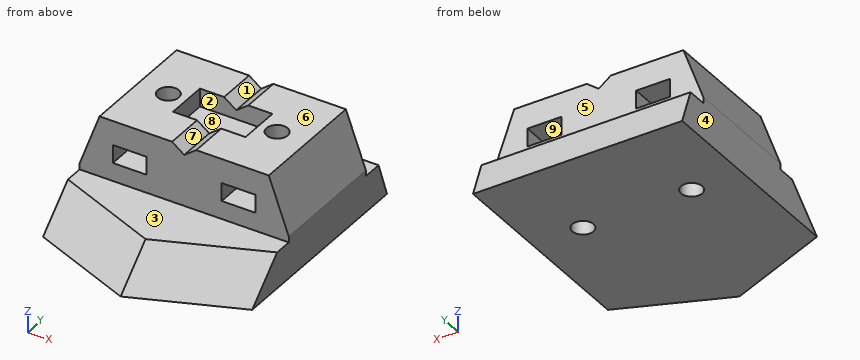
```python
from build123d import *

# Parameters (mm, degrees)
ESBO_O1_W                = 34.6
ESBO_O1_H                = 26
RESSALTO_EXTRUS_O1_DEPTH = 7
ESBO_O10_W               = 34.6
ESBO_O10_H               = 2.5
RESSALTO_EXTRUS_O4_DEPTH = 7
CHANFRO1_SIZE            = 7
CHANFRO2_SIZE2           = 7
CHANFRO2_SIZE            = 2.54779164
ESBO_O11_W               = 5.6
ESBO_O11_H               = 3
RESSALTO_EXTRUS_O5_DEPTH = 10
ESBO_O12_R               = 1.75
CORTE_EXTRUS_O1_DEPTH    = 20
ESBO_O13_W               = 34.6
ESBO_O13_H               = 5.5
ESBO_O13_H_2             = 18.393079324
CORTE_EXTRUS_O2_DEPTH    = 1
ESBO_O14_W               = 12
ESBO_O14_H               = 7
CORTE_EXTRUS_O3_DEPTH    = 3


with BuildPart() as part:
    # Esboço1 → Ressalto-extrusão1 (new body)
    with BuildSketch(Plane.XY):
        Rectangle(ESBO_O1_W, ESBO_O1_H)
    extrude(amount=RESSALTO_EXTRUS_O1_DEPTH)

    # Esboço10 → Ressalto-extrusão4 (add)
    with BuildSketch(Plane(origin=(0, 0, 0), x_dir=(-1, 0, 0), z_dir=(0, 0, -1))):
        Polygon((-17.3, -19.5), (0, -26.5), (17.3, -19.5), (17.3, -13), (-17.3, -13), align=None)
        with Locations((0, 14.25)):
            Rectangle(ESBO_O10_W, ESBO_O10_H)
    extrude(amount=-RESSALTO_EXTRUS_O4_DEPTH)

    # Chanfro1
    chanfro1_edges = [part.edges().sort_by_distance(p)[0] for p in [
        (8.65, -23, 7),
        (-8.65, -23, 7),
    ]]
    chamfer(chanfro1_edges, length=CHANFRO1_SIZE - 0.0001)  # a hair under: the kernel refuses the full size

    # Chanfro2
    chanfro2_edges = [part.edges().sort_by_distance(p)[0] for p in [
        (0, 15.5, 7),
    ]]
    chanfro2_side = [part.faces().sort_by_distance(p)[0] for p in [
        (0, 15.449044167, 7),
    ]]
    chamfer(chanfro2_edges, length=CHANFRO2_SIZE - 0.0001, length2=CHANFRO2_SIZE2 - 0.0001, reference=chanfro2_side[0])  # a hair under: the kernel refuses the full size

    # Esboço11 → Ressalto-extrusão5 (add, symmetric)
    with BuildSketch(Plane(origin=(0, 0, 0), x_dir=(1, 0, 0), z_dir=(0, 1, 0))):
        Polygon((-17.3, -7), (-14, -16), (-2, -16), (0, -14.5), (2, -16), (14, -16), (17.3, -7), align=None)
        with Locations((-9, -10.5)):
            Rectangle(ESBO_O11_W, ESBO_O11_H, mode=Mode.SUBTRACT)
        with Locations((9, -10.5)):
            Rectangle(ESBO_O11_W, ESBO_O11_H, mode=Mode.SUBTRACT)
    extrude(amount=RESSALTO_EXTRUS_O5_DEPTH, both=True)

    # Esboço12 → Corte-extrusão1 (cut)
    with BuildSketch(Plane.XY.offset(16)):
        with Locations((-9, 0)):
            Circle(ESBO_O12_R)
        with Locations(Location((9, 0, 0), (0, 0, 180))):
            Circle(ESBO_O12_R)
    extrude(amount=-CORTE_EXTRUS_O1_DEPTH, mode=Mode.SUBTRACT)

    # Esboço13 → Corte-extrusão2 (cut)
    with BuildSketch(Plane.XY.offset(7)):
        with Locations((0, 12.75)):
            Rectangle(ESBO_O13_W, ESBO_O13_H)
        with Locations((0, -19.196539662)):
            Rectangle(ESBO_O13_W, ESBO_O13_H_2)
    extrude(amount=-CORTE_EXTRUS_O2_DEPTH, mode=Mode.SUBTRACT)

    # Esboço14 → Corte-extrusão3 (cut)
    with BuildSketch(Plane.XY.offset(16)):
        Rectangle(ESBO_O14_W, ESBO_O14_H)
    extrude(amount=-CORTE_EXTRUS_O3_DEPTH, mode=Mode.SUBTRACT)


solid = part.part
```
Geometry check sheet. Reference: the model listing, model coordinates, mm. Face numbers are marked on the shaded views. A direction names the side the tool comes from. Coordinates: 2 decimals unless noted, no trailing zeros. Order: outer loops, then holes, each group sorted by start corner. A loop starts at its lowest first (then second) coordinate and runs counter-clockwise, first axis right, second up. Notation, with made-up numbers: (7, 39) - (64, 39) arc R20 cw to (64, 44) - close; hole circle Ø10 at (-2.75, 74). An arc over 180 degrees is marked (long way). Answer in a Markdown table with one row per item. Add a question column.
1. Section check C-C (z = 2.5). Enter the section's corners in (x, y), plus the area to 3 significant figures.
2. Section check A-A (y = -9.5). Enter the section's corners in (x, z).
3. Material ranges on L1, parallel to Y at x = 9, z = 7; L2, parallel to X at y = -8, z = 11; L3, parallel to Z at x = 2, y = -1.5, recorded low to high. Write a range as [from, to].
4. Access from +Z, -Z, +X, -X, +Y, -Y to the whole of each face (thin tool, end or side, straight path). Record for the marked faces 5, 6, 7, 8 and 9.
5. Gauge pin test, flat ends, axial feed: pin 1 Ø3.5 at (y, z) = (4, 10.5) entering from +X; pin 2 Ø3 at (x, y) = (-9, 0) entering from +Z; pin 3 Ø3 at (x, y) = (-9.5, -1) entering from +Z; pin 4 Ø3.5 at (x, z) = (0.5, 14) entering from +Y. Record the tip position at first contact, or that the pin passes through.
6. Draft check along X on the marked faces 1, 2, 3 and 4. Enter one of: +X half, -X half, draft (parallel to the pull), parting line (faces both ways), or undercut.
7. Section check B-B (x = -9). Give the number of separate pieces and of enclosed holes in the cut face, plus the area to 3 significant figures.
Data:
| question | item | result |
|---|---|---|
| 1 | outline | (-17.3, -16.8) - (0, -23.8) - (17.3, -16.8) - (17.3, 14.59) - (-17.3, 14.59) - close; hole circle Ø3.5 at (-9, 0); hole circle Ø3.5 at (9, 0) |
| 1 | area | 1,190 mm² |
| 2 | outline | (-17.3, 0) - (17.3, 0) - (17.3, 7) - (14, 16) - (2, 16) - (0, 14.5) - (-2, 16) - (-14, 16) - (-17.3, 7) - close; hole (-11.8, 9) - (-6.2, 9) - (-6.2, 12) - (-11.8, 12) - close; hole (6.2, 9) - (11.8, 9) - (11.8, 12) - (6.2, 12) - close |
| 3 | L1 | y = [-10, -1.75], [1.75, 10] |
| 3 | L2 | x = [-15.83, -11.8], [-6.2, 6.2], [11.8, 15.83] |
| 3 | L3 | z = [0, 13] |
| 4 | face 5 | +Z, +X, -X, +Y |
| 4 | face 6 | +Z, +X, -X, +Y, -Y |
| 4 | face 7 | +Z, +Y, -Y |
| 4 | face 8 | +Z |
| 4 | face 9 | +Y, -Y |
| 5 | pin 1 | stops at x = 16.66 |
| 5 | pin 2 | passes through |
| 5 | pin 3 | stops at z = 16 |
| 5 | pin 4 | stops at y = 10 |
| 6 | face 1 | undercut |
| 6 | face 2 | undercut |
| 6 | face 3 | draft |
| 6 | face 4 | -X half |
| 7 | separate pieces | 4 |
| 7 | enclosed holes | 0 |
| 7 | area | 299 mm² |
